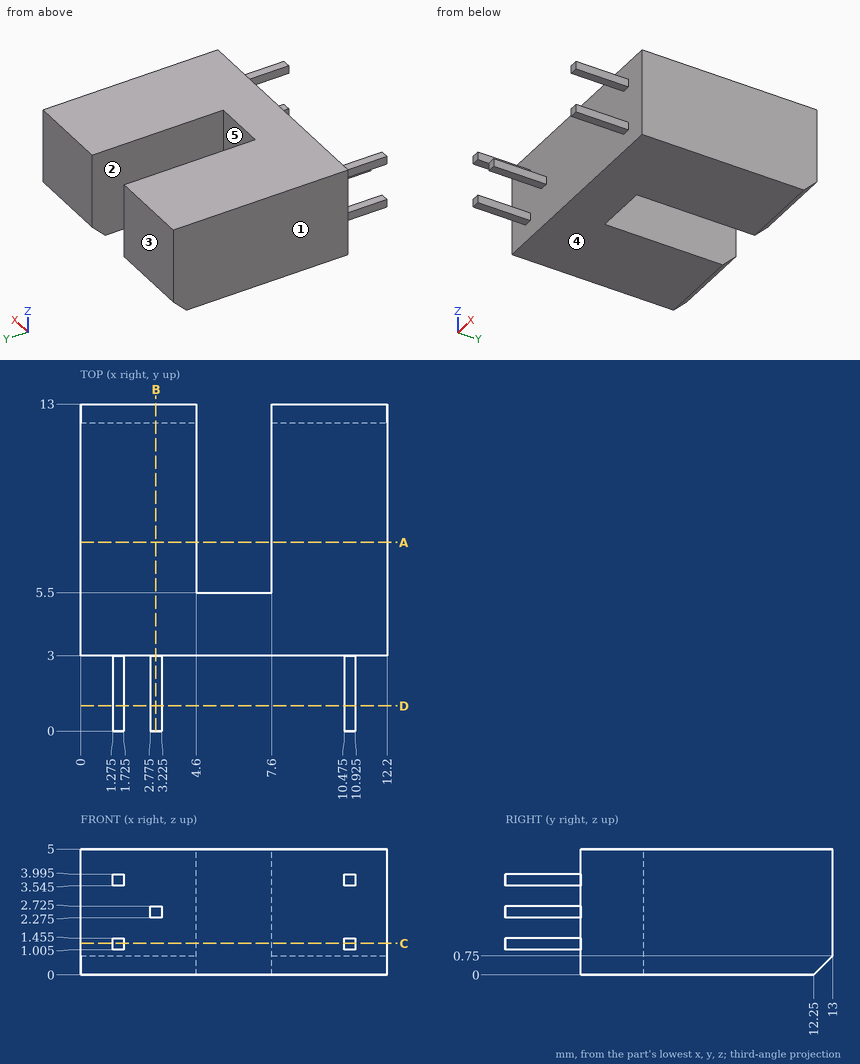
Input: dimensioned drawing with shaded views. Units: mm. Origin: part minimum x, y, z. A direction names the side the tool comes from. Coordinates: 2 decimals unless noted, no trailing zeros. Loops run counter-clockwise (first coordinate to the right, second up) from the corner with the lowest first, then second, coordinate; pieces in that order, holes last. Notation, with made-up numbers: (75, 2) -> (114, 2) arc R22 ccw to (114, 25) -> close; hole circle Ø1 at (50, 62). An arc over 180 degrees is marked (long way). Use a Markdown table: item, result. Add a question column.
(1) Access query for the marked faces 4 and 5. Directions: +Z, -Z, +X, -X, +Y, -Y. A direction counts if a zero-diameter tool reaches every point of the face in a straight line with its end or side. Return the directions, or none.
(2) Pin query (flat end, axial travel): pin 1 Ø0.5 at (y, z) = (1.5, 1.5) entering from +X (3 decimals); pin 2 Ø2 at (x, z) = (5, 2.5) entering from -Y; pin 3 Ø0.5 at (x, y) = (1.5, 1) entering from -Z (3 decimals). Return the tip coordinate at first contact, or that it passes through.
(3) Section query A-A, the plane y = 7.5. Return loops of the section in (x, z), plus the area to 3 significant figures.
(4) Line query: line 1 along X through (y, z) = (8, 0.4); line 2 along Y through (x, z) = (7.5, 0.85); line 3 along Y through (x, z) = (0.75, 1.1). Output: solid intervals per line, ascending.
(5) Section query D-D, the plane y = 1. Return loops of the section in (x, z) (3 decimals), plus the area to 3 significant figures.
(6) Section query B-B, the plane x = 3. Return loops of the section in (y, z) (3 decimals).
(7) Mould query, pull axis X, two halves, no side actions, for the marked faces 1, 2 and 3. Classes: pulls with the +X half, pulls with the -X half, needs draft (parallel to the pull), parting line crosses it, or undercut.
(8) Section query C-C, the plane z = 1.25. Return loops of the section in (x, y) (3 decimals).
Answer:
| question | item | result |
|---|---|---|
| 1 | face 4 | -Z, +X, -X, +Y, -Y |
| 1 | face 5 | +Z, -Z, +Y |
| 2 | pin 1 | stops at x = 10.925 |
| 2 | pin 2 | stops at y = 3 |
| 2 | pin 3 | stops at z = 1.005 |
| 3 | outline | (0, 0) -> (4.6, 0) -> (4.6, 5) -> (0, 5) -> close; (7.6, 0) -> (12.2, 0) -> (12.2, 5) -> (7.6, 5) -> close |
| 3 | area | 46.0 mm^2 |
| 4 | line 1 | x = 0 to 4.6, 7.6 to 12.2 |
| 4 | line 2 | y = 3 to 5.5 |
| 4 | line 3 | y = 3 to 13 |
| 5 | outline | (1.275, 1.005) -> (1.725, 1.005) -> (1.725, 1.455) -> (1.275, 1.455) -> close; (1.275, 3.545) -> (1.725, 3.545) -> (1.725, 3.995) -> (1.275, 3.995) -> close; (2.775, 2.275) -> (3.225, 2.275) -> (3.225, 2.725) -> (2.775, 2.725) -> close; (10.475, 1.005) -> (10.925, 1.005) -> (10.925, 1.455) -> (10.475, 1.455) -> close; (10.475, 3.545) -> (10.925, 3.545) -> (10.925, 3.995) -> (10.475, 3.995) -> close |
| 5 | area | 1.01 mm^2 |
| 6 | outline | (0, 2.275) -> (3, 2.275) -> (3, 0) -> (12.25, 0) -> (13, 0.75) -> (13, 5) -> (3, 5) -> (3, 2.725) -> (0, 2.725) -> close |
| 7 | face 1 | pulls with the -X half |
| 7 | face 2 | undercut |
| 7 | face 3 | needs draft |
| 8 | outline | (0, 3) -> (1.275, 3) -> (1.275, 0) -> (1.725, 0) -> (1.725, 3) -> (10.475, 3) -> (10.475, 0) -> (10.925, 0) -> (10.925, 3) -> (12.2, 3) -> (12.2, 13) -> (7.6, 13) -> (7.6, 5.5) -> (4.6, 5.5) -> (4.6, 13) -> (0, 13) -> close |
